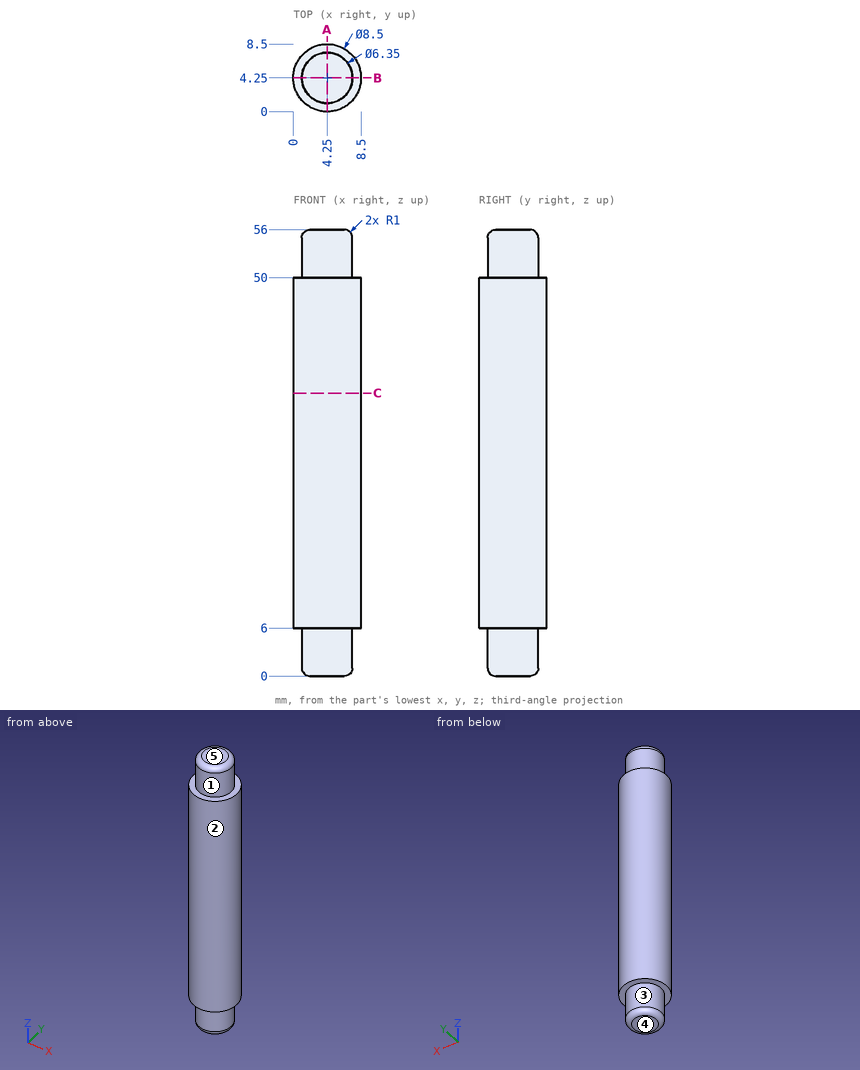
Answer from the drawing. Dimensions are ordinates in mm from the lowest x, y and z of the part. A direction names the side the tool comes from. Round coordinates to 2 decimals unless told otherwise and drop trailing zeros. Write each loop counter-clockwise with the first axis right and the second up, starting at its lowest first coordinate (ties: lowest second). Pieces come first, ordered by that corner, then holes.
1. Straight lines are drawn through the part: L1, parallel to Y at x = 4.5, z = 6.5; L2, parallel to Z at x = 7.5, y = 2; L3, parallel to Z at x = 4.75, y = 2. For each, find the intervals that lie inside material, in ascending order.
2. Which of the six approach directions +Z, -Z, +X, -X, +Y, -Y give full straight-line access (tool end or side, diameter ignored) to the marked faces 1 and 2?
3. The part is cut by section C-C, the plane z = 35.5. Determine the outline of the cut face in (x, y), then the cut area to 3 significant figures.
4. The part is cut by section A-A, the plane x = 4.25. Determine the outline of the cut face in (y, z) (3 decimals), then the cut area to 3 significant figures.
5. Determine the mould class of the marked faces 3, 4 and 5 for opening direction Z: pulls with the +Z half, pulls with the -Z half, needs draft (parallel to the pull), parting line crosses it, or undercut.
6. Given pin 1 Ø4 at (x, z) = (2, 34) entering from +Y; pin 2 Ø3 at (y, z) = (7, 11) entering from +X; pin 3 Ø1 at (x, y) = (7.5, 5) entering from -Z, each flat-ended and moving along its own axis, determine where each tip first touches the part or whether it passes through.
Values:
1. L1: y = 0.01 to 8.49
1. L2: z = 6 to 50
1. L3: z = 0.01 to 55.99
2. face 1: +Z
2. face 2: +Z, -Z
3. outline: circle Ø8.5 at (4.25, 4.25)
3. area: 56.7 mm2
4. outline: (0, 6) - (1.075, 6) - (1.075, 1) arc R1 ccw to (2.075, 0) - (6.425, 0) arc R1 ccw to (7.425, 1) - (7.425, 6) - (8.5, 6) - (8.5, 50) - (7.425, 50) - (7.425, 55) arc R1 ccw to (6.425, 56) - (2.075, 56) arc R1 ccw to (1.075, 55) - (1.075, 50) - (0, 50) - close
4. area: 449 mm2
5. face 3: needs draft
5. face 4: pulls with the -Z half
5. face 5: pulls with the +Z half
6. pin 1: stops at y = 8.49
6. pin 2: stops at x = 8.31
6. pin 3: stops at z = 0.25
